```python
from build123d import *

# Parameters (mm, degrees)
BOSS_EXTRUDE1_DEPTH      = 8
BOSS_EXTRUDE1_TAPER      = 19.700000000000042
FILLET1_R                = 1
SHELL1_T                 = -1.5
BOSS_EXTRUDE2_REACH      = 16.924
BOSS_EXTRUDE2_END_RADIUS = 41.49999999999999
SKETCH4_R                = 2.75
SKETCH4_R_2              = 2
CUT_EXTRUDE2_REACH       = 16.924
CUT_EXTRUDE2_END_RADIUS  = 41.49999999999999
BOSS_EXTRUDE3_START      = -1.43836
SKETCH8_W                = 12.593266454489342
SKETCH8_H                = 12.593266454489337
BOSS_EXTRUDE3_DEPTH      = 1.43836


with BuildPart() as part:
    # Sketch1 → Boss-Extrude1 (new body)
    with BuildSketch(Plane(origin=(0, 0, 0), x_dir=(1, 0, 0), z_dir=(0, 1, 0))):
        Polygon((8.999999999999996, 9.000000000000002), (-9.000000000000004, 8.999999999999998), (-9, -9.000000000000002), (9, -9), align=None)
    extrude(amount=BOSS_EXTRUDE1_DEPTH, taper=BOSS_EXTRUDE1_TAPER)

    # Sketch3 → Cut-Revolve2 (revolve, cut)
    with BuildSketch(Plane(origin=(0, 0, 0), x_dir=(-0.7071067811865476, 0, -0.7071067811865476), z_dir=(0.7071067811865476, 0, -0.7071067811865476))):
        with BuildLine():
            Line((-40, 47.04752471069329), (40, 47.04752471069329))
            ThreePointArc((40, 47.04752471069329), (-7.35e-15, 7.047524710693288), (-40, 47.04752471069329))
        make_face()
    revolve(axis=Axis((28.2842712474619, 47.04752471069329, 28.2842712474619), (-0.7071067811865476, 0, -0.7071067811865476)), mode=Mode.SUBTRACT)

    # Fillet1
    fillet1_edges = [part.edges().sort_by_distance(p)[0] for p in [
        (-3.7925e-13, 7.546443435071887, 6.297982062276191),
        (6.297982062276188, 7.546443435071887, 3.606e-13),
        (-6.297982062276191, 7.5464434350718905, -3.5616e-13),
        (3.7481e-13, 7.546443435071887, -6.297982062276189),
        (7.567792650420588, 4, 7.567792650420591),
        (7.5677926504205875, 4, -7.567792650420591),
        (-7.567792650420594, 4, -7.567792650420589),
        (-7.567792650420591, 4, 7.567792650420593),
    ]]
    fillet(fillet1_edges, radius=FILLET1_R)

    # Shell1
    shell1_openings = [part.faces().sort_by_distance(p)[0] for p in [
        (0, 0, 0),
    ]]
    offset(amount=SHELL1_T, openings=shell1_openings)

    # Boss-Extrude2: up to this sphere (the profile starts outside it)
    boss_extrude2_end = Location((0, 47.04752471069329, 0)) * Sphere(BOSS_EXTRUDE2_END_RADIUS, mode=Mode.PRIVATE)
    # Sketch4 → Boss-Extrude2 (add, up to the surface)
    with BuildSketch(Plane.XZ, mode=Mode.PRIVATE) as boss_extrude2_sk1:
        with Locations(Location((0, 0, 0), (0, 0, 270))):
            Circle(SKETCH4_R)
        Circle(SKETCH4_R_2, mode=Mode.SUBTRACT)
    boss_extrude2_tool1 = extrude(boss_extrude2_sk1.sketch, amount=-BOSS_EXTRUDE2_REACH, mode=Mode.PRIVATE) - boss_extrude2_end
    add(boss_extrude2_tool1.solids().sort_by_distance((0, 0, 2.672218))[0])
    # Sketch4 → Boss-Extrude2 (add, up to the surface)
    with BuildSketch(Plane.XZ, mode=Mode.PRIVATE) as boss_extrude2_sk2:
        Circle(SKETCH4_R_2)
    boss_extrude2_tool2 = extrude(boss_extrude2_sk2.sketch, amount=-BOSS_EXTRUDE2_REACH, mode=Mode.PRIVATE) - boss_extrude2_end
    add(boss_extrude2_tool2.solids().sort_by_distance((0, 0, 0))[0])

    # Cut-Extrude2: up to this sphere (the profile starts outside it)
    cut_extrude2_end = Location((0, 47.04752471069329, 0)) * Sphere(CUT_EXTRUDE2_END_RADIUS, mode=Mode.PRIVATE)
    # Sketch6 → Cut-Extrude2 (cut, up to the surface)
    with BuildSketch(Plane.XZ, mode=Mode.PRIVATE) as cut_extrude2_sk1:
        Polygon((-1.1e-16, -2.05), (-0.5500000000000002, -2.05), (-0.5500000000000002, -0.5500000000000002), (-2.05, -0.5500000000000005), (-2.05, -4.3e-16), (-2.05, 0.5499999999999996), (-0.5500000000000002, 0.5499999999999997), (-0.5500000000000002, 2.0499999999999994), (-1.1e-16, 2.0499999999999994), (0.5500000000000002, 2.0499999999999994), (0.5500000000000002, 0.5499999999999997), (2.05, 0.55), (2.0499999999999994, -2.1e-16), (2.05, -0.55), (0.55, -0.55), (0.5499999999999999, -2.0499999999999994), align=None)
    cut_extrude2_tool1 = extrude(cut_extrude2_sk1.sketch, amount=-CUT_EXTRUDE2_REACH, mode=Mode.PRIVATE) - cut_extrude2_end
    add(cut_extrude2_tool1.solids().sort_by_distance((0, 0, 0))[0], mode=Mode.SUBTRACT)

    # Sketch8 → Boss-Extrude3 (add)
    with BuildSketch(Plane(origin=(0, 4.7625, 0), x_dir=(-1, 0, 0), z_dir=(0, -1, 0)).offset(BOSS_EXTRUDE3_START)):
        Rectangle(SKETCH8_W, SKETCH8_H)
    extrude(amount=BOSS_EXTRUDE3_DEPTH)


solid = part.part
```
Could you check a few things on this model? Use its own coordinates, in mm. A direction names the side the tool comes from. Round coordinates to 2 decimals unless told otherwise and drop trailing zeros.
Q1. For P1, Ø1.7, axis at y = 1.5, z = 1.5, coming from the -X side; P2, Ø0.6, axis at x = 0, y = 3, coming from the +Z side; P3, Ø0.8, axis at x = -1.5, y = 1.5, coming from the +Z side; P4, Ø8, axis at x = -1.5, z = 0, coming from the -Y side, each with a flat end and sliding along its axis, tell me the tip position at first contact or that it passes through.
Q2. Please list where these lines run through material, in increasing order: L1, parallel to Z at x = -0.25, y = 4; L2, parallel to Z at x = -3.75, y = 0.5; L3, parallel to Z at x = -0.25, y = 2.5.
Q3. I want a section at A-A (y = 2). Give the number of separate pieces and of enclosed holes in the cut face, and give its area (3 significant figures).
Q4. On a 3-axis mill with a long thin cutter (end or side, diameter ignored), from which of +Z, -Z, +X, -X, +Y, -Y can I reach the whole of each face in a straight line? I mean faces 1 (the flat face through (0, 0, 8)), 2 (the flat face through (1, 4.762, -3)). Say none if no direction works.
Q5. Thinking about a two-plate mould opening in Z: for faces 3 (the flat face through (-1, 2, -0.55)), 4 (the flat face through (1, 0, -1)), which applies, pulls with the +Z half, pulls with the -Z half, needs draft (parallel to the pull), parting line crosses it, or undercut?
Answer below:
1. P1: stops at x = -8.77
1. P2: stops at z = 8.03
1. P3: stops at z = 8.61
1. P4: stops at y = 0
2. L1: z = -7.57 to -5.97, -2.74 to -2.05, 2.05 to 2.74, 5.97 to 7.57
2. L2: z = -8.82 to -7.23, 7.23 to 8.82
2. L3: z = -8.1 to -6.51, -2.74 to -2.05, 2.05 to 2.74, 6.51 to 8.1
3. separate pieces: 2
3. enclosed holes: 2
3. area: 111 mm2
4. face 1: +Z, -Z, +X, -X, -Y
4. face 2: -Y
5. face 3: undercut
5. face 4: needs draft
